Job drawing, mm, ordinate dimensions from the low corner. One solid piece. A direction names the side the tool comes from. Round coordinates to 2 decimals unless told otherwise and drop trailing zeros. Loops run counter-clockwise (first coordinate to the right, second up) from the corner with the lowest first, then second, coordinate; pieces in that order, holes last.
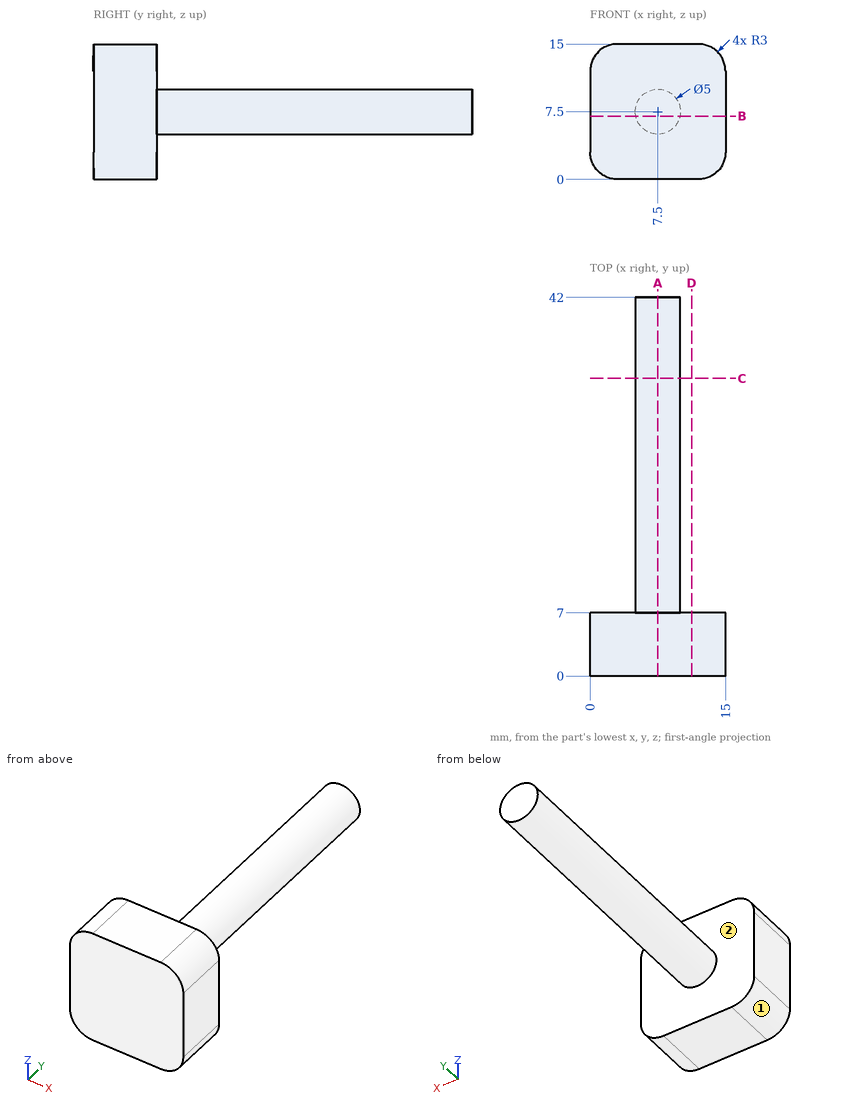
Item 1: Flat gauge pins, fed straight in: P1, Ø6, axis at x = 10, z = 8, coming from the +Y side; P2, Ø5, axis at x = 7, y = 13.5, coming from the -Z side; P3, Ø8, axis at y = 31.5, z = 10, coming from the -X side; P4, Ø1.5, axis at x = 10.5, z = 9, coming from the +Y side. Where does each tip first touch, or does it go through?
Answers follow:
P1: stops at y = 42
P2: stops at z = 5
P3: stops at x = 5
P4: stops at y = 7
Item 2: Cut at A-A, the plane x = 7.5. Give the cut face in (y, z), plus the area to 3 significant figures.
Answers follow:
outline: (0, 0) - (7, 0) - (7, 5) - (42, 5) - (42, 10) - (7, 10) - (7, 15) - (0, 15) - close
area: 280 mm2
Item 3: Cut at B-B, the plane z = 7. Give the cut face in (x, y), plus the area to 3 significant figures.
Answers follow:
outline: (0, 0) - (15, 0) - (15, 7) - (9.95, 7) - (9.95, 42) - (5.05, 42) - (5.05, 7) - (0, 7) - close
area: 276 mm2
Item 4: Probe line 1 (Y direction, x = 5.5, z = 11.5); line 2 (Z direction, x = 9, y = 28); line 3 (Z direction, x = 7, y = 8.5). List the from-to ranges inside material, lowest first.
Answers follow:
line 1: y = 0 to 7
line 2: z = 5.5 to 9.5
line 3: z = 5.05 to 9.95
Item 5: Cut at D-D, the plane x = 11.25. Give the cut face in (y, z), plus the area to 3 significant figures.
Answers follow:
outline: (0, 0) - (7, 0) - (7, 15) - (0, 15) - close
area: 105 mm2
Item 6: Cut at C-C, the plane y = 33. Give the cut face in (x, z), plus the area to 3 significant figures.
Answers follow:
outline: circle Ø5 at (7.5, 7.5)
area: 19.6 mm2
Item 7: 3-axis set-ups, long thin cutter, end or side, ignore diameter. For the marked faces 1 and 2: which of +Z, -Z, +X, -X, +Y, -Y reach the whole face in a straight line?
Answers follow:
face 1: -Z, -X, +Y, -Y
face 2: +Y
